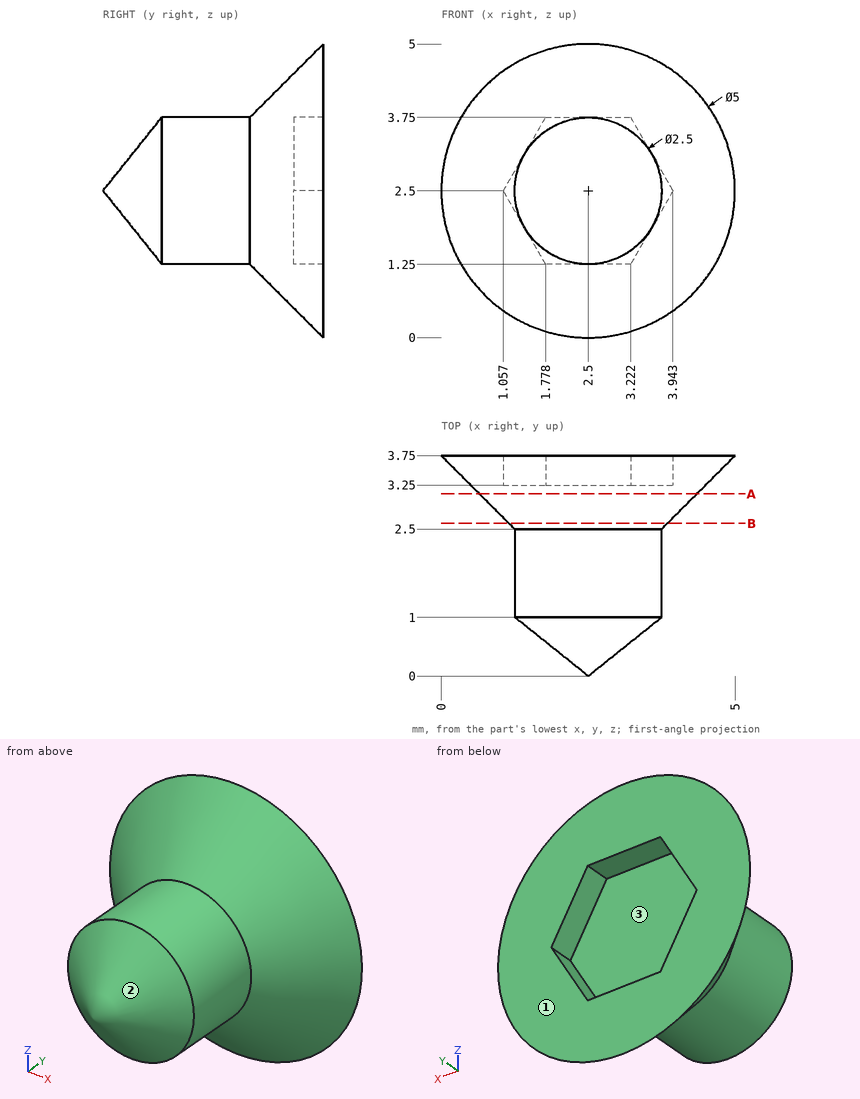
Check sheet for the drawn part. Datum: minimum x, y, z corner. Units: mm. Round coordinates to 2 decimals unless told otherwise and drop trailing zeros. Order: outer loops, then holes, each group sorted by start corner. A loop starts at its lowest first (then second) coordinate and runs counter-clockwise, first axis right, second up.
1) Section check A-A (y = 3.1). Record the boundary of the cut face in (x, z).
2) Go/stop test with flat-tipped pins: pin 1 Ø1 at (y, z) = (2, 3.5) entering from -X (1 decimal); pin 2 Ø1 at (x, y) = (3, 1.5) entering from +Z. Record where each tip stops, or that it passes through.
3) Section check B-B (y = 2.6). Record the boundary of the cut face in (x, z).
4) Scan lines: line 1 (X direction, y = 3.65, z = 3.65) (1 decimal); line 2 (Y direction, x = 1.3, z = 4.1); line 3 (X direction, y = 1.8, z = 3.55). Record each from-to range of solid material in increasing order.
5) Mould release check, pull along X, two halves, no side actions. Record for the marked faces 1, 2 and 3: +X half, -X half, draft (parallel to the pull), parting line (faces both ways), or undercut.
Result:
1. outline: circle Ø3.7 at (2.5, 2.5)
2. pin 1: stops at x = 1.4
2. pin 2: stops at z = 3.75
3. outline: circle Ø2.7 at (2.5, 2.5)
4. line 1: x = 0.4 to 1.7, 3.3 to 4.6
4. line 2: y = 3.25 to 3.75
4. line 3: x = 1.82 to 3.18
5. face 1: draft
5. face 2: parting line
5. face 3: undercut
